Geometry check sheet. Reference: the model listing, model coordinates, mm. Face numbers are marked on the shaded views. A direction names the side the tool comes from. Give positions to 0.01 mm unless a question says otherwise; leave off trailing zeros. Write each loop counter-clockwise with the first axis right and the second up, starting at its lowest first coordinate (ties: lowest second). Pieces come first, ordered by that corner, then holes. Notation, with made-up numbers: (43, 71.5) -> (47, 71.5) arc R21 cw to (47, 79.5) -> close; hole circle Ø11 at (63.25, -1). An arc over 180 degrees is marked (long way). Write item = value, one per line. Start each with the question number.
1. Thickness scan on line 1 along Z through (x, y) = (32.5, 0); line 2 along Y through (x, z) = (12, -5) (3 decimals); line 3 along X through (y, z) = (8.75, -2.75). Record the ranges inside material, lowest first.
2. Set-up check for the marked faces 1 and 2: record each of +Z, -Z, +X, -X, +Y, -Y from which the full face is reachable in a straight line by a thin tool's end or side.
3. Cross-section at C-C, the plane z = 0. Record the cut outline in (x, y) (3 decimals).
4. Mould release check, pull along Y, two halves, no side actions. Record for the marked faces 3, 4 and 5: pulls with the +Y half, pulls with the -Y half, needs draft (parallel to the pull), parting line crosses it, or undercut.
5. Cross-section at D-D, the plane y = 0. Record the cut outline in (x, z).
6. Depth check by flat-ended pin: P1, Ø3, axis at x = 5.5, z = -2, coming from the -Y side; P2, Ø5, axis at x = 21.5, y = 8.5, coming from the -Z side; P3, Ø7, axis at y = 0, z = 0, coming from the -X side. Enter the tip coordinate at first touch or a pass-through.
7. Cross-section at B-B, the plane y = 15.5. Record the cut outline in (x, z).
8. Cross-section at A-A, the plane x = 5.5. Record the cut outline in (y, z) (3 decimals), plus the area to 3 significant figures.
```python
from build123d import *

# Parameters (mm, degrees)
BOSS_EXTRUDE1_DEPTH = 40
SKETCH2_W           = 40
SKETCH2_H           = 16
BOSS_EXTRUDE2_DEPTH = 12
FILLET1_R           = 1


with BuildPart() as part:
    # Sketch1 → Boss-Extrude1 (new body)
    with BuildSketch(Plane(origin=(0, 0, 0), x_dir=(0, 0, -1), z_dir=(1, 0, 0))):
        with BuildLine():
            Line((-3.625, -1.690968657), (-3.625, -3.041889066))
            Line((-3.625, -3.041889066), (-6, -3.041889066))
            Line((-6, -3.041889066), (-6, 6))
            Line((-6, 6), (6, 6))
            Line((6, 6), (6, -3.041889066))
            Line((6, -3.041889066), (3.625, -3.041889066))
            Line((3.625, -3.041889066), (3.625, -1.690968657))
            ThreePointArc((3.625, -1.690968657), (0, 4), (-3.625, -1.690968657))
        make_face()
    extrude(amount=BOSS_EXTRUDE1_DEPTH)

    # Sketch2 → Boss-Extrude2 (add)
    with BuildSketch(Plane.XY.offset(6)):
        with Locations((20, 14)):
            Rectangle(SKETCH2_W, SKETCH2_H)
        Polygon((8.5, 17), (8.5, 19.125), (31.5, 19.125), (31.5, 7.125), (8.5, 7.125), (8.5, 11), (4.5, 11), (4.5, 17), align=None, mode=Mode.SUBTRACT)
    extrude(amount=-BOSS_EXTRUDE2_DEPTH)

    # Fillet1
    fillet1_edges = [part.edges().sort_by_distance(p)[0] for p in [
        (40, 9.479055467, -6),
        (40, 22, 0),
        (0, 22, 0),
        (20, 22, 6),
        (20, 22, -6),
        (40, 9.479055467, 6),
        (0, 9.479055467, 6),
        (0, 9.479055467, -6),
    ]]
    fillet(fillet1_edges, radius=FILLET1_R)


solid = part.part
```
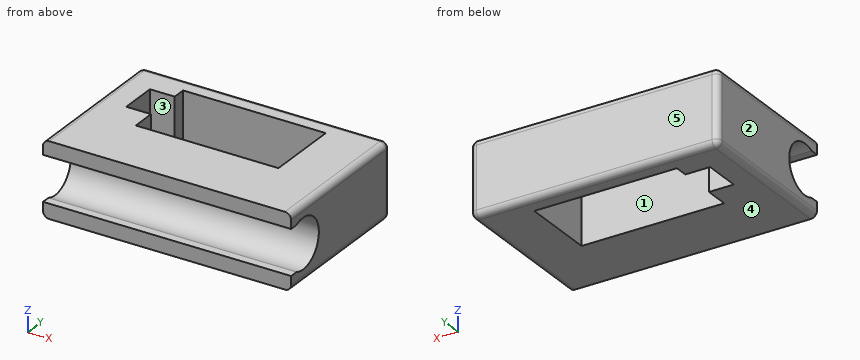
Answers:
q1.line_1 = -6 to -4, 4 to 6
q1.line_2 = -3.042 to 7.125, 19.125 to 22
q1.line_3 = 0 to 8.5, 31.5 to 40
q2.face_1 = +Z, -Z
q2.face_2 = +Z, -Z, -X, +Y, -Y
q3.outline = (0, 4) -> (40, 4) -> (40, 21) arc R1 ccw to (39, 22) -> (1, 22) arc R1 ccw to (0, 21) -> close; hole (4.5, 11) -> (8.5, 11) -> (8.5, 7.125) -> (31.5, 7.125) -> (31.5, 19.125) -> (8.5, 19.125) -> (8.5, 17) -> (4.5, 17) -> close
q4.face_3 = undercut
q4.face_4 = needs draft
q4.face_5 = pulls with the +Y half
q5.outline = (0, -5) arc R1 ccw to (1, -6) -> (39, -6) arc R1 ccw to (40, -5) -> (40, -4) -> (0, -4) -> close; (0, 4) -> (40, 4) -> (40, 5) arc R1 ccw to (39, 6) -> (1, 6) arc R1 ccw to (0, 5) -> close
q6.P1 = 1.94
q6.P2 = -6
q6.P3 = through
q7.outline = (0, -5) arc R1 ccw to (1, -6) -> (4.5, -6) -> (4.5, 6) -> (1, 6) arc R1 ccw to (0, 5) -> close; (31.5, -6) -> (39, -6) arc R1 ccw to (40, -5) -> (40, 5) arc R1 ccw to (39, 6) -> (31.5, 6) -> close
q8.outline = (-3.042, -6) -> (11, -6) -> (11, 6) -> (-3.042, 6) -> (-3.042, 3.625) -> (-1.691, 3.625) arc R4 cw (long way) to (-1.691, -3.625) -> (-3.042, -3.625) -> close; (17, -6) -> (21, -6) arc R1 ccw to (22, -5) -> (22, 5) arc R1 ccw to (21, 6) -> (17, 6) -> close
q8.area = 180 mm^2
